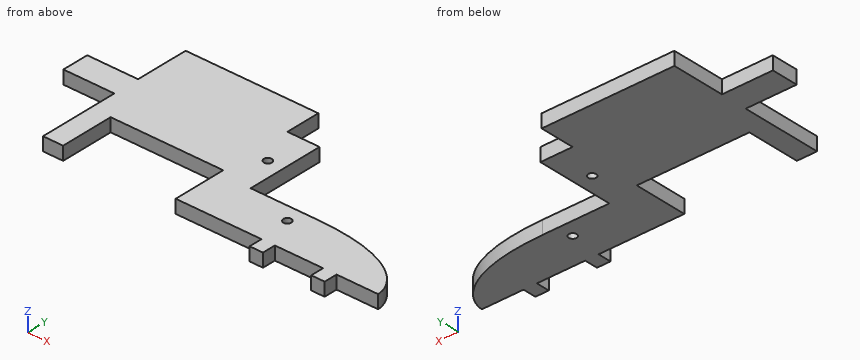
from build123d import *

# Parameters (mm, degrees)
ESQUISSE1_R             = 1.5
BOSS_EXTRU_1_DEPTH      = 5
BOSS_EXTRU_2_DEPTH      = 5
ESQUISSE3_W             = 236.288260714
ESQUISSE3_H             = 122.224262112
ENL_V_MAT_EXTRU_1_DEPTH = 5


with BuildPart() as part:
    # Esquisse1 → Boss.-Extru.1 (new body)
    with BuildSketch(Plane.XY):
        Polygon((0, 0), (32, 0), (32, -5), (37, -5), (37, 0), (37, 18), (12, 18), (12, 47), (0, 47), align=None)
        with Locations((6, 32)):
            Circle(ESQUISSE1_R, mode=Mode.SUBTRACT)
        with Locations((31, 12)):
            Circle(ESQUISSE1_R, mode=Mode.SUBTRACT)
    extrude(amount=BOSS_EXTRU_1_DEPTH)

    # Esquisse2 → Boss.-Extru.2 (add)
    with BuildSketch(Plane(origin=(0, 0, 0), x_dir=(-1, 0, 0), z_dir=(0, 0, -1))):
        with BuildLine():
            Line((-37, 0), (-55, 0))
            Line((-55, 0), (-55, -5))
            Line((-55, -5), (-60, -5))
            Line((-60, -5), (-60, 0))
            Line((-60, 0), (-75.5, 0))
            add(Edge.make_bspline(
                [(-75.5, 0), (-75.5, 5.982232529), (-67.685409636, 18), (-37, 18)],
                knots=[0, 0, 0, 0, 1, 1, 1, 1], degree=3))
            Line((-37, 18), (-37, 0))
        make_face()
        Polygon((42, 0), (49.5, 0), (49.5, 30), (68.5, 30), (68.5, 40), (49.5, 40), (49.5, 110), (68.5, 110), (68.5, 120), (49.5, 120), (49.5, 142), (-1, 142), (-1, 167), (-10, 167), (-10, 172), (-20, 172), (-20, 167), (-25, 167), (-25, 90), (20, 90), (20, 60), (0, 60), (0, 20), (42, 20), align=None)
    extrude(amount=-BOSS_EXTRU_2_DEPTH)

    # Esquisse3 → Enlèv. mat.-Extru.1 (cut)
    with BuildSketch(Plane(origin=(0, 0, 0), x_dir=(-1, 0, 0), z_dir=(0, 0, -1))):
        with Locations((68.98963671, 121.112131056)):
            Rectangle(ESQUISSE3_W, ESQUISSE3_H)
    extrude(amount=-ENL_V_MAT_EXTRU_1_DEPTH, mode=Mode.SUBTRACT)


solid = part.part
The listing builds one solid part. Answer for the finished solid, in the listing's coordinates (mm). Coordinates: 2 decimals unless noted, no trailing zeros. Write each loop counter-clockwise with the first axis right and the second up, starting at its lowest first coordinate (ties: lowest second). Pieces come first, ordered by that corner, then holes. Notation, with made-up numbers: (28.5, 86) - (37.5, 86) arc R20 ccw to (37.5, 118) - close; hole circle Ø11 at (40, 31.5). An arc over 180 degrees is marked (long way). Answer as CSV lines item,"result".
1. Straight lines are drawn through the part: line 1 (Y direction, x = 6, z = 1.25); line 2 (X direction, y = 27, z = 4.55); line 3 (Y direction, x = -32, z = 2.6). For each, find the intervals that lie inside material, in ascending order. Write a range as [from, to].
Computed values:
line 1,"y = [0, 30.5], [33.5, 47]"
line 2,"x = [-49.5, 12]"
line 3,"y = [20, 60]"
2. Find section B-B (y = 32). Give the vertices of the cut face in (x, z).
Computed values:
outline,"(-68.5, 0) - (4.5, 0) - (4.5, 5) - (-68.5, 5) - close; (7.5, 0) - (12, 0) - (12, 5) - (7.5, 5) - close"
3. Find section D-D (x = -20). Give the vertices of the cut face in (y, z), plus the area to 3 significant figures.
Computed values:
outline,"(20, 0) - (60, 0) - (60, 5) - (20, 5) - close"
area,"200 mm²"
4. Given P1, Ø2.5, axis at x = 6.5, z = 1.5, coming from the +Y side; P2, Ø1.5, axis at y = 52.5, z = 1.5, coming from the +X side; P3, Ø2, axis at x = -25.5, z = 2.5, coming from the -Y side; P4, Ø1.8, axis at x = 6, y = 32, coming from the +Z side, each flat-ended and moving along its own axis, determine where each tip first touches the part or whether it passes through.
Computed values:
P1,"stops at y = 47"
P2,"stops at x = 0"
P3,"stops at y = 20"
P4,"passes through"
5. Find section A-A (x = 6). Give the vertices of the cut face in (y, z).
Computed values:
outline,"(0, 0) - (30.5, 0) - (30.5, 5) - (0, 5) - close; (33.5, 0) - (47, 0) - (47, 5) - (33.5, 5) - close"
6. Find section C-C (z = 0.9). Give the number of separate pieces and of enclosed holes in the cut face, plus the area to 3 significant figures.
Computed values:
separate pieces,"1"
enclosed holes,"2"
area,"3,920 mm²"
